Design review of the part built by this model. Coordinates are the model's own, in mm. A direction names the side the tool comes from. Give positions to 0.01 mm unless a question says otherwise; leave off trailing zeros. Order: outer loops, then holes, each group sorted by start corner. A loop starts at its lowest first (then second) coordinate and runs counter-clockwise, first axis right, second up.
```python
from build123d import *

# Parameters (mm, degrees)
SALIENTE_EXTRUIR1_START   = -2.75
SALIENTE_EXTRUIR1_DEPTH   = 5.5
SALIENTE_EXTRUIR1_2_DEPTH = 2.75
SALIENTE_EXTRUIR2_DEPTH   = 38
SALIENTE_EXTRUIR3_START   = 2.75
SALIENTE_EXTRUIR3_DEPTH   = 2.75
CROQUIS4_W                = 23
CROQUIS4_H                = 43.5
CORTAR_EXTRUIR1_DEPTH     = 8.25
CORTAR_EXTRUIR2_DEPTH     = 2.75
CROQUIS6_W                = 38
CROQUIS6_H                = 22.249999999
CORTAR_EXTRUIR3_DEPTH     = 16.59246817
CROQUIS7_W                = 3.203765914
CROQUIS7_H                = 38
CORTAR_EXTRUIR4_DEPTH     = 8.25
CROQUIS8_W                = 3.203765916
CROQUIS8_H                = 38
CORTAR_EXTRUIR5_DEPTH     = 8.25
CROQUIS9_W                = 14
CROQUIS9_H                = 38
CORTAR_EXTRUIR6_DEPTH     = 0.703765915
CROQUIS10_W               = 14
CROQUIS10_H               = 38
CORTAR_EXTRUIR7_DEPTH     = 0.703765915
SALIENTE_EXTRUIR4_START   = 2.75
SALIENTE_EXTRUIR4_DEPTH   = 2.75
CORTAR_EXTRUIR8_DEPTH     = 2.75
CROQUIS13_W               = 12.249999999
CROQUIS13_H               = 2.75
CORTAR_EXTRUIR9_DEPTH     = 74.034358614
CROQUIS14_W               = 12.249999999
CROQUIS14_H               = 2.75
CORTAR_EXTRUIR10_DEPTH    = 74.034358614
CROQUIS15_W               = 5
CROQUIS15_H               = 2.75
CROQUIS16_W               = 5
CROQUIS16_H               = 2.75
TALADRO1_D                = 10.15
TALADRO1_DEPTH            = 2.75
TALADRO2_D                = 10.15
CORTAR_EXTRUIR11_REACH    = 202.135
SALIENTE_EXTRUIR5_DEPTH   = 2.75
SALIENTE_EXTRUIR6_START   = -2.75
SALIENTE_EXTRUIR6_DEPTH   = 2.75
CROQUIS24_W               = 27.125
CROQUIS24_H               = 38
SALIENTE_EXTRUIR7_DEPTH   = 2.5
CROQUIS25_R               = 2
CORTAR_EXTRUIR12_DEPTH    = 2.5


with BuildPart() as part:
    # Saliente-Extruir1: read off the stored shape, not the designer's step
    # Saliente-Extruir1 outline → Saliente-Extruir1 (new body)
    with BuildSketch(Plane(origin=(0, 40.75, 0), x_dir=(-1, 0, 0), z_dir=(0, 1, 0)).offset(SALIENTE_EXTRUIR1_START)):
        with BuildLine():
            Line((161.177139208, 19.345694485), (182.584423689, 27.755698719))
            Line((182.584423689, 27.755698719), (171.432026769, 56.143619441))
            ThreePointArc((171.432026769, 56.143619441), (156.523382412, 62.642259564), (150.024742289, 47.733615207))
            Line((150.024742289, 47.733615207), (161.177139208, 19.345694485))
        make_face()
    extrude(amount=SALIENTE_EXTRUIR1_DEPTH)

    # Saliente-Extruir1 2 outline → Saliente-Extruir1 2 (add)
    with BuildSketch(Plane(origin=(0, 40.75, 0), x_dir=(-1, 0, 0), z_dir=(0, 1, 0))):
        with BuildLine():
            ThreePointArc((161.177139208, 19.345694485), (176.085783565, 12.847054362), (182.584423687, 27.755698719))
            Line((182.584423687, 27.755698719), (161.177139208, 19.345694485))
        make_face()
    extrude(amount=SALIENTE_EXTRUIR1_2_DEPTH)

    # Croquis2 → Saliente-Extruir2 (add)
    with BuildSketch(Plane.XZ.offset(-38)):
        Polygon((-171.432026768, 56.143619442), (-150.024742288, 47.733615205), (-161.177139209, 19.345694483), (-182.584423689, 27.755698719), align=None)
    extrude(amount=SALIENTE_EXTRUIR2_DEPTH)

    # Croquis3 → Saliente-Extruir3 (add)
    with BuildSketch(Plane.XZ.offset(SALIENTE_EXTRUIR3_START)):
        with BuildLine():
            Line((-182.584423688, 27.755698719), (-171.432026768, 56.143619441))
            ThreePointArc((-171.432026768, 56.143619441), (-156.523382412, 62.642259564), (-150.024742289, 47.733615207))
            Line((-150.024742289, 47.733615207), (-161.177139208, 19.345694485))
            Line((-161.177139208, 19.345694485), (-182.584423688, 27.755698719))
        make_face()
    extrude(amount=-SALIENTE_EXTRUIR3_DEPTH)

    # Croquis4 → Cortar-Extruir1 (cut)
    with BuildSketch(Plane(origin=(-14.965700114, 0, -38.094511116), x_dir=(-0.9307514991056489, 0, 0.3656523580022251), z_dir=(-0.3656523580022251, 0, -0.9307514991056489))):
        with Locations((168.589662745, 19)):
            Rectangle(CROQUIS4_W, CROQUIS4_H)
    extrude(amount=-CORTAR_EXTRUIR1_DEPTH, mode=Mode.SUBTRACT)

    # Croquis5 → Cortar-Extruir2 (cut)
    with BuildSketch(Plane(origin=(0, 40.75, 0), x_dir=(1, 0, 0), z_dir=(0, 1, 0))):
        with BuildLine():
            Line((-161.142417183, -28.195858914), (-176.585881806, -34.262934025))
            ThreePointArc((-176.585881806, -34.262934025), (-167.602648859, -34.440489141), (-161.142417183, -28.195858914))
        make_face()
    extrude(amount=-CORTAR_EXTRUIR2_DEPTH, mode=Mode.SUBTRACT)

    # Croquis6 → Cortar-Extruir3 (cut)
    with BuildSketch(Plane(origin=(-149.193349022, 0, 58.611670162), x_dir=(0, 1, 0), z_dir=(0.9307514991056486, 0, -0.3656523580022258))):
        with Locations((19, -21.553766865)):
            Rectangle(CROQUIS6_W, CROQUIS6_H)
    extrude(amount=-CORTAR_EXTRUIR3_DEPTH, mode=Mode.SUBTRACT)

    # Croquis7 → Cortar-Extruir4 (cut)
    with BuildSketch(Plane(origin=(-3.8133032, 0, -9.706590403), x_dir=(0.9307514990825102, 0, -0.36565235806112356), z_dir=(0.36565235806112356, 0, 0.9307514990825102))):
        with Locations((-158.691545702, 19)):
            Rectangle(CROQUIS7_W, CROQUIS7_H)
    extrude(amount=-CORTAR_EXTRUIR4_DEPTH, mode=Mode.SUBTRACT)

    # Croquis8 → Cortar-Extruir5 (cut)
    with BuildSketch(Plane(origin=(-3.8133032, 0, -9.706590403), x_dir=(0.9307514990825102, 0, -0.36565235806112356), z_dir=(0.36565235806112356, 0, 0.9307514990825102))):
        with Locations((-178.487779787, 19)):
            Rectangle(CROQUIS8_W, CROQUIS8_H)
    extrude(amount=-CORTAR_EXTRUIR5_DEPTH, mode=Mode.SUBTRACT)

    # Croquis9 → Cortar-Extruir6 (cut)
    with BuildSketch(Plane(origin=(-164.636813645, 0, 64.678745273), x_dir=(-0.3656523580022247, 0, -0.930751499105649), z_dir=(0.930751499105649, 1.4355340193330324e-15, -0.3656523580022247))):
        with Locations((25.678766864, 19)):
            Rectangle(CROQUIS9_W, CROQUIS9_H)
    extrude(amount=-CORTAR_EXTRUIR6_DEPTH, mode=Mode.SUBTRACT)

    # Croquis10 → Cortar-Extruir7 (cut)
    with BuildSketch(Plane(origin=(-149.193349022, 0, 58.611670162), x_dir=(0.3656523580022248, 0, 0.930751499105649), z_dir=(-0.930751499105649, -1.4355340193330322e-15, 0.3656523580022248))):
        with Locations((-25.678766864, 19)):
            Rectangle(CROQUIS10_W, CROQUIS10_H)
    extrude(amount=-CORTAR_EXTRUIR7_DEPTH, mode=Mode.SUBTRACT)

    # Croquis11 → Saliente-Extruir4 (add)
    with BuildSketch(Plane.XZ.offset(2.75).offset(SALIENTE_EXTRUIR4_START)):
        with BuildLine():
            Line((-150.024742289, 47.733615207), (-161.177139208, 19.345694485))
            ThreePointArc((-161.177139208, 19.345694485), (-176.085783565, 12.847054362), (-182.584423687, 27.755698719))
            Line((-182.584423687, 27.755698719), (-171.432026769, 56.143619441))
            ThreePointArc((-171.432026769, 56.143619441), (-156.523382412, 62.642259564), (-150.024742289, 47.733615207))
        make_face()
    extrude(amount=-SALIENTE_EXTRUIR4_DEPTH)

    # Croquis12 → Cortar-Extruir8 (cut)
    with BuildSketch(Plane(origin=(0, 0, 0), x_dir=(-1, 0, 0), z_dir=(0, 1, 0))):
        with BuildLine():
            Line((161.142417183, 28.195858914), (176.585881806, 34.262934025))
            ThreePointArc((176.585881806, 34.262934025), (167.602648859, 34.440489141), (161.142417183, 28.195858914))
        make_face()
    extrude(amount=-CORTAR_EXTRUIR8_DEPTH, mode=Mode.SUBTRACT)

    # Croquis13 → Cortar-Extruir9 (cut, through all)
    with BuildSketch(Plane(origin=(-146.211439094, 0, 57.440205601), x_dir=(-0.36565235800222584, 0, -0.9307514991056486), z_dir=(0.9307514991056486, 0, -0.36565235800222584))):
        with Locations((16.553766864, -4.125)):
            Rectangle(CROQUIS13_W, CROQUIS13_H)
    extrude(amount=-CORTAR_EXTRUIR9_DEPTH, mode=Mode.SUBTRACT)

    # Croquis14 → Cortar-Extruir10 (cut, through all)
    with BuildSketch(Plane(origin=(-146.211439094, 0, 57.440205601), x_dir=(-0.36565235800222584, 0, -0.9307514991056486), z_dir=(0.9307514991056486, 0, -0.36565235800222584))):
        with Locations((16.553766864, 42.125)):
            Rectangle(CROQUIS14_W, CROQUIS14_H)
    extrude(amount=-CORTAR_EXTRUIR10_DEPTH, mode=Mode.SUBTRACT)

    # Croquis15 → Revolución1 (revolve)
    with BuildSketch(Plane(origin=(0, 0, 51.938617325), x_dir=(-1, 0, 0), z_dir=(0, 0, -1))):
        with Locations((158.228384529, -4.125)):
            Rectangle(CROQUIS15_W, CROQUIS15_H)
    revolve(axis=Axis((-160.728384529, -5.5, 51.938617325), (0, 1, 0)))

    # Croquis16 → Revolución2 (revolve)
    with BuildSketch(Plane(origin=(0, 0, 51.938617325), x_dir=(-1, 0, 0), z_dir=(0, 0, -1))):
        with Locations((158.228384529, 42.125)):
            Rectangle(CROQUIS16_W, CROQUIS16_H)
    revolve(axis=Axis((-160.728384529, 40.75, 51.938617325), (0, 1, 0)))

    # Taladro1
    with Locations(Plane(origin=(0, -5.5, 0), x_dir=(-1, 0, 0), z_dir=(0, -1, 0))):
        with Locations((171.880781448, -23.550696602)):
            Hole(TALADRO1_D / 2, depth=TALADRO1_DEPTH)

    # Taladro2 (through all)
    with Locations(Plane(origin=(0, 40.75, 0), x_dir=(-1, 0, 0), z_dir=(0, -1, 0))):
        with Locations((171.880781448, -23.550696602)):
            Hole(TALADRO2_D / 2)

    # Cortar-Extruir11: up to this face of the body (flat: up to its plane)
    cortar_extruir11_end = Plane(part.part.faces().sort_by_distance((-169.996704911, 43.5, 28.346528005))[0])
    # Croquis21 → Cortar-Extruir11 (cut, up to the picked face)
    with BuildSketch(Plane.XZ.offset(5.5), mode=Mode.PRIVATE) as cortar_extruir11_sk1:
        Polygon((-173.671647461, 50.44276651), (-152.264362982, 42.032762276), (-144.951315822, 60.647792258), (-166.358600301, 69.057796492), align=None)
    cortar_extruir11_tool1 = split(extrude(cortar_extruir11_sk1.sketch, amount=-CORTAR_EXTRUIR11_REACH, mode=Mode.PRIVATE), bisect_by=cortar_extruir11_end, keep=Keep.BOTH, mode=Mode.PRIVATE)
    add(cortar_extruir11_tool1.solids().sort_by(Axis((-159.311482, -5.5, 55.545279), (0, 1, 0)))[0], mode=Mode.SUBTRACT)

    # Croquis22 → Saliente-Extruir5 (add)
    with BuildSketch(Plane.XZ.offset(2.75)):
        Polygon((-152.264362982, 42.032762276), (-173.671647461, 50.44276651), (-164.530338511, 73.711553987), (-158.015078017, 71.151987481), align=None)
    extrude(amount=-SALIENTE_EXTRUIR5_DEPTH)

    # Croquis23 → Saliente-Extruir6 (add)
    with BuildSketch(Plane(origin=(0, 40.75, 0), x_dir=(1, 0, 0), z_dir=(0, 1, 0)).offset(SALIENTE_EXTRUIR6_START)):
        Polygon((-158.015078017, -71.151987481), (-152.264362982, -42.032762276), (-173.671647461, -50.44276651), (-164.530338511, -73.711553987), align=None)
    extrude(amount=SALIENTE_EXTRUIR6_DEPTH)

    # Croquis24 → Saliente-Extruir7 (add)
    with BuildSketch(Plane(origin=(-167.618723573, 0, 65.850209835), x_dir=(0.36565235800222584, 0, 0.9307514991056486), z_dir=(-0.9307514991056486, 0, 0.36565235800222584))):
        with Locations((-5.116266864, 19)):
            Rectangle(CROQUIS24_W, CROQUIS24_H)
    extrude(amount=-SALIENTE_EXTRUIR7_DEPTH)

    # Croquis25 → Cortar-Extruir12 (cut)
    with BuildSketch(Plane(origin=(-167.618723573, 0, 65.850209835), x_dir=(0.36565235800222584, 0, 0.9307514991056486), z_dir=(-0.9307514991056486, 0, 0.36565235800222584))):
        with Locations((-0.866266864, 6.5)):
            Circle(CROQUIS25_R)
        with Locations((-0.866266864, 31.5)):
            Circle(CROQUIS25_R)
        with Locations((-13.366266864, 19)):
            Circle(CROQUIS25_R)
    extrude(amount=-CORTAR_EXTRUIR12_DEPTH, mode=Mode.SUBTRACT)


solid = part.part
```
1. For pin 1 (7 mm diameter, centred on x = -168, z = 47, fed in from -Y); pin 2 (2 mm diameter, centred on y = 12.5, z = 52.5, fed in from +X); pin 3 (4 mm diameter, centred on y = 8.5, z = 47.5, fed in from +X), all flat-tipped, find the tip position at first contact; note any pin that passes through.
Recorded:
pin 1: stops at y = -2.75
pin 2: stops at x = -169.78
pin 3: stops at x = -171.36
2. Take a section at B-B (y = -2). State the section outline as (x, z) points.
Recorded:
outline: (-179.57, 35.43) - (-176.59, 34.26) arc R11.7 cw to (-161.14, 28.2) - (-158.16, 27.02) - (-152.26, 42.03) - (-158.02, 71.15) - (-164.53, 73.71) - close
3. Machinability: for faces 5 (the face through (-167.723, -1.356, 34.487)), 6 (the face through (-165.06, -4.14, 40.48)), 7 (the face through (-162, 38, 50)), 8 (the face through (-162, 40.75, 55)), 9 (the face through (-159.3, 19.3, 27.47)), which of the approach directions +Z, -Z, +X, -X, +Y, -Y give a long, thin tool a straight path to every point of the face, cutting with its end or side? Answer none if there is none.
Recorded:
face 5: -Z
face 6: +Z, +X, -Y
face 7: none
face 8: +Z, +X, +Y
face 9: -Z, -X
4. Take a section at C-C (x = -171). State how many separate pieces and enclosed holes the cut face has, then the cut area to 3 significant figures.
Recorded:
separate pieces: 3
enclosed holes: 1
area: 481 mm2
5. For line 1 along Y through (x, z) = (-165.5, 63); line 2 along Y through (x, z) = (-173, 40.5); line 3 along Y through (x, z) = (-155.5, 40), list the stretches that pass through material, from the lowest coordinate up.
Recorded:
line 1: y = -2.75 to 0, 38 to 40.75
line 2: y = -5.5 to 0, 38 to 43.5
line 3: y = -2.75 to 40.75
6. Take a section at A-A (y = 12). State the section outline as (x, z) points.
Recorded:
outline: (-179.57, 35.43) - (-177.24, 34.52) - (-162.2, 72.8) - (-164.53, 73.71) - close; (-160.49, 27.94) - (-158.16, 27.02) - (-153.04, 40.05) - (-155.37, 40.97) - close
7. Draft analysis for pull direction X (two halves, no side actions). For faces 1 (the face through (-169, 43.5, 29)), 2 (the face through (-175.849, -4.144, 12.757)), 3 (the face through (-157.964, 19.266, 34.363)), 4 (the face through (-162, 0, 51)), state which applies: pulls with the +X half, pulls with the -X half, needs draft (parallel to the pull), parting line crosses it, or undercut.
Recorded:
face 1: needs draft
face 2: parting line crosses it
face 3: undercut
face 4: undercut
